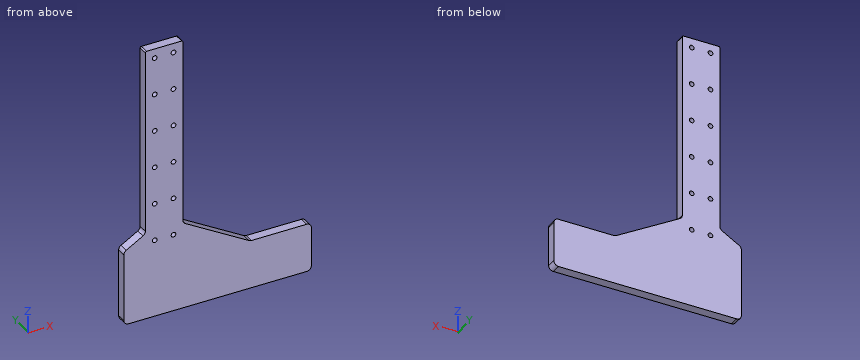
from build123d import *

# Parameters (mm, degrees)
F0_R     = 3.175
F1_DEPTH = 6.35


with BuildPart() as f1:
    # F0 (on Front) → F1 (new body, symmetric)
    with BuildSketch(Plane.XZ):
        with BuildLine():
            Line((23.8125, 0), (-23.8125, 0))
            ThreePointArc((-23.8125, 0), (-24.935032, -0.464968), (-25.4, -1.5875))
            Line((-25.4, -1.5875), (-25.4, -250.333826))
            ThreePointArc((-25.4, -250.333826), (-26.250739, -253.508826), (-28.575, -255.833087))
            Line((-28.575, -255.833087), (-51.373449, -268.995778))
            ThreePointArc((-51.373449, -268.995778), (-53.697711, -271.320039), (-54.548449, -274.495039))
            Line((-54.548449, -274.495039), (-54.548449, -366.078865))
            ThreePointArc((-54.548449, -366.078865), (-52.688577, -370.568993), (-48.198449, -372.428865))
            Line((-48.198449, -372.428865), (193.101551, -372.428865))
            ThreePointArc((193.101551, -372.428865), (197.591679, -370.568993), (199.451551, -366.078865))
            Line((199.451551, -366.078865), (199.451551, -312.994769))
            ThreePointArc((199.451551, -312.994769), (197.591679, -308.504641), (193.101551, -306.644769))
            Line((193.101551, -306.644769), (118.284892, -306.644769))
            ThreePointArc((118.284892, -306.644769), (116.641391, -306.428398), (115.109892, -305.79403))
            Line((115.109892, -305.79403), (28.575, -255.833087))
            ThreePointArc((28.575, -255.833087), (26.250739, -253.508826), (25.4, -250.333826))
            Line((25.4, -250.333826), (25.4, -1.5875))
            ThreePointArc((25.4, -1.5875), (24.935032, -0.464968), (23.8125, 0))
        make_face()
        with Locations((-12.7, -266.7)):
            Circle(F0_R, mode=Mode.SUBTRACT)
        with Locations((-12.7, -215.9)):
            Circle(F0_R, mode=Mode.SUBTRACT)
        with Locations((12.7, -266.7)):
            Circle(F0_R, mode=Mode.SUBTRACT)
        with Locations((12.7, -215.9)):
            Circle(F0_R, mode=Mode.SUBTRACT)
        with Locations((-12.7, -165.1)):
            Circle(F0_R, mode=Mode.SUBTRACT)
        with Locations((-12.7, -114.3)):
            Circle(F0_R, mode=Mode.SUBTRACT)
        with Locations((12.7, -165.1)):
            Circle(F0_R, mode=Mode.SUBTRACT)
        with Locations((12.7, -114.3)):
            Circle(F0_R, mode=Mode.SUBTRACT)
        with Locations((-12.7, -63.5)):
            Circle(F0_R, mode=Mode.SUBTRACT)
        with Locations((-12.7, -12.7)):
            Circle(F0_R, mode=Mode.SUBTRACT)
        with Locations((12.7, -63.5)):
            Circle(F0_R, mode=Mode.SUBTRACT)
        with Locations((12.7, -12.7)):
            Circle(F0_R, mode=Mode.SUBTRACT)
    extrude(amount=F1_DEPTH, both=True)


solid = f1.part
Here's how the part is built. I have some questions about the finished solid (model axes, mm). Round coordinates to 2 decimals unless told otherwise and drop trailing zeros. Loops run counter-clockwise (first coordinate to the right, second up) from the corner with the lowest first, then second, coordinate; pieces in that order, holes last. Notation, with made-up numbers: M 18.25,-10.5 L 72.25,-10.5 A18 ccw 72.25,23.5 Z; hole C 80,42 d2. An arc over 180 degrees is marked long. Write each question's results on one line, items separated by ' | '. Start each with the question number.
(1) I want a section at A-A (y = 3). State how many separate pieces and enclosed holes the cut face has, then the cut area to 3 significant figures.
(2) I want a section at C-C (z = -281.5). Please give me the cut outline in (x, y), then the cut area to 3 significant figures.
(3) If I drill on probe 1 along X at (y, z) = (3.5, -215.9) (3 decimals); probe 2 along X at (y, z) = (3.5, -266.7) (3 decimals); probe 3 along Z at (x, y) = (149, -1), over which ranges is the centre line in solid material (lowest first)? Write a range as from..to.
(4) Will these pins go through, and if not, where does the flat tip stop? P1, Ø5.5, axis at x = 12.7, z = -114.3, coming from the -Y side; P2, Ø3, axis at x = 86, y = -2, coming from the +Z side; P3, Ø4, axis at x = 160, y = -1, coming from the +Z side; P4, Ø1, axis at y = 4, z = -102, coming from the -X side.
(5) I want a section at B-B (x = 165.5). Please give me the cut outline in (y, z).
Solved:
1) separate pieces: 1 | enclosed holes: 12 | area: 35,600 mm²
2) outline: M -54.55,-6.35 L 73.03,-6.35 L 73.03,6.35 L -54.55,6.35 Z | area: 1,620 mm²
3) probe 1: x = -25.4..-15.875, -9.525..9.525, 15.875..25.4 | probe 2: x = -47.397..-15.875, -9.525..9.525, 15.875..47.397 | probe 3: z = -372.43..-306.64
4) P1: passes through | P2: stops at z = -288.12 | P3: stops at z = -306.64 | P4: stops at x = -25.4
5) outline: M -6.35,-372.43 L 6.35,-372.43 L 6.35,-306.64 L -6.35,-306.64 Z
